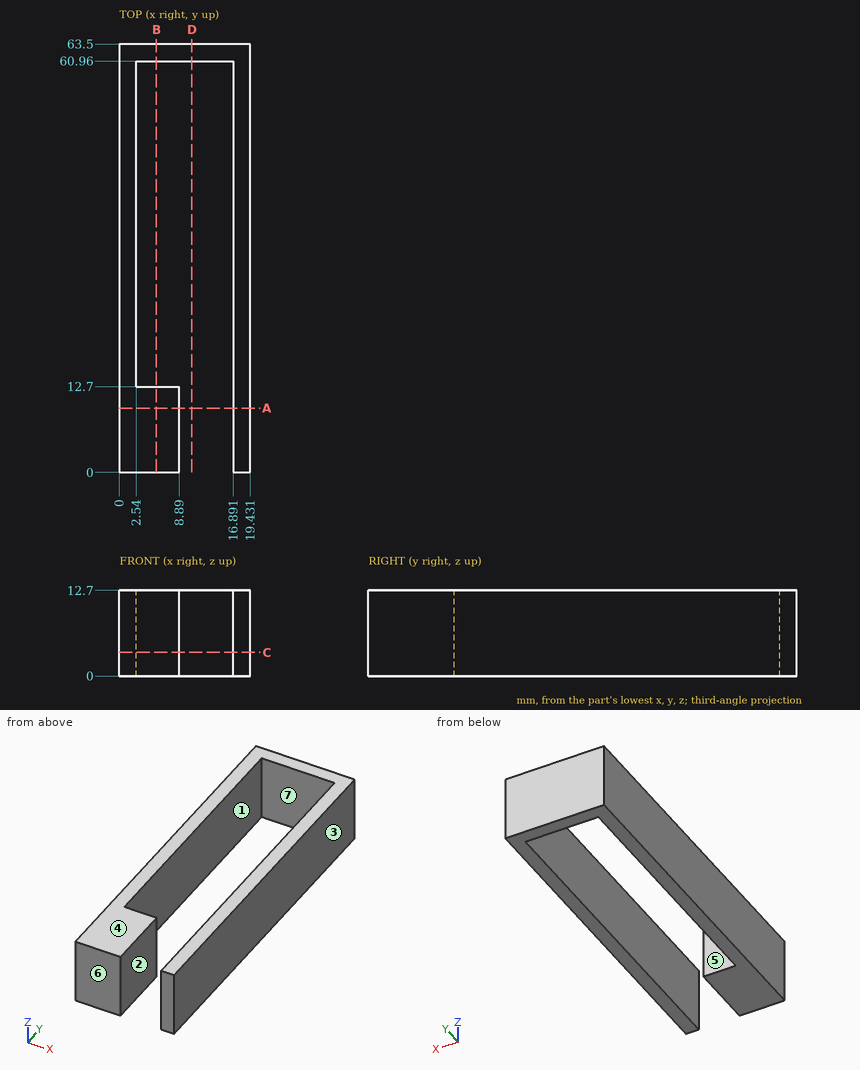
For this review, use the dimensioned drawing (mm, ordinates from the lowest corner) and the shaded views. A direction names the side the tool comes from. Coordinates: 2 decimals unless noted, no trailing zeros. Loops run counter-clockwise (first coordinate to the right, second up) from the corner with the lowest first, then second, coordinate; pieces in that order, holes last. Notation, with made-up numbers: (1, 6.5) -> (27, 6.5) arc R27 ccw to (27, 44.5) -> close; hole circle Ø5 at (21, 62). An arc over 180 degrees is marked (long way). Return JSON: item names as keys, results as strings. Group by question number.
(1) Consider section D-D, the plane x = 10.75. Give the boundary of the cut face in (y, z).
(2) Consider section B-B, the plane x = 5.5. Give the boundary of the cut face in (y, z), plus the area to 3 significant figures.
(3) Mouldability with a two-part tool opening along Y and no side actions: class the marked faces 4, 5, 6 and 7 as pulls with the +Y half, pulls with the -Y half, needs draft (parallel to the pull), parting line crosses it, or undercut.
(4) Consider section A-A, the plane y = 9.5. Give the boundary of the cut face in (x, z).
(5) To check wall thickness, follow L1, parallel to Y at x = 4.5, z = 3.5; L2, parallel to X at y = 9.5, z = 4.75; L3, parallel to X at y = 16.5, z = 5.75. State the ranges of each line that lie inside material, in increasing order.
(6) Tool access review of the marked faces 1, 2 and 3: name each direction out of +Z, -Z, +X, -X, +Y, -Y from which nothing blocks a thin tool from reaching the whole face with its end or side.
(7) Consider section C-C, the plane z = 3.5. Give the boundary of the cut face in (x, y).
(8) For pin 1 Ø2 at (y, z) = (12, 1.5) entering from -X; pin 2 Ø8 at (x, y) = (9.5, 43) entering from -Z, all flat-tipped, find the tip position at first contact; note any pin that passes through.
Results below:
{
 "1": {"outline": "(60.96, 0) -> (63.5, 0) -> (63.5, 12.7) -> (60.96, 12.7) -> close"},
 "2": {"outline": "(0, 0) -> (12.7, 0) -> (12.7, 12.7) -> (0, 12.7) -> close; (60.96, 0) -> (63.5, 0) -> (63.5, 12.7) -> (60.96, 12.7) -> close", "area": "194 mm2"},
 "3": {"face 4": "needs draft", "face 5": "undercut", "face 6": "pulls with the -Y half", "face 7": "undercut"},
 "4": {"outline": "(0, 0) -> (8.89, 0) -> (8.89, 12.7) -> (0, 12.7) -> close; (16.89, 0) -> (19.43, 0) -> (19.43, 12.7) -> (16.89, 12.7) -> close"},
 "5": {"L1": "y = 0 to 12.7, 60.96 to 63.5", "L2": "x = 0 to 8.89, 16.89 to 19.43", "L3": "x = 0 to 2.54, 16.89 to 19.43"},
 "6": {"face 1": "+Z, -Z", "face 2": "+Z, -Z, -Y", "face 3": "+Z, -Z, +X, +Y, -Y"},
 "7": {"outline": "(0, 0) -> (8.89, 0) -> (8.89, 12.7) -> (2.54, 12.7) -> (2.54, 60.96) -> (16.89, 60.96) -> (16.89, 0) -> (19.43, 0) -> (19.43, 63.5) -> (0, 63.5) -> close"},
 "8": {"pin 1": "stops at x = 0", "pin 2": "passes through"}
}
